```python
from build123d import *

# Parameters (mm, degrees)
F1_DEPTH = 15
F2_R     = 37.5
F3_DEPTH = 50
F4_R     = 7.5
F5_DEPTH = 40
F7_DEPTH = 50


with BuildPart() as f1:
    # F0 (on Front) → F1 (new body, symmetric)
    with BuildSketch(Plane.XZ):
        Polygon((-25, 200), (-75, 200), (-17.5, -30), (15, -30), (187.5, 200), (112.5, 200), (9.375, 62.5), align=None)
    extrude(amount=F1_DEPTH, both=True)

    # F2 (on Front) → F3 (join, symmetric)
    with BuildSketch(Plane.XZ):
        Circle(F2_R)
    extrude(amount=F3_DEPTH, both=True)

    # F4 (on face) → F5 (join)
    with BuildSketch(Plane.XZ.offset(50)):
        Circle(F4_R)
    extrude(amount=F5_DEPTH)

    # F6 (on Top) → F7 (cut, symmetric)
    with BuildSketch(Plane.XY):
        Polygon((-20, -79.282032), (-20, -90), (20, -90), align=None)
    extrude(amount=F7_DEPTH, both=True, mode=Mode.SUBTRACT)


solid = f1.part
```
Build history of the part. All positions in model axes, mm. A direction names the side the tool comes from. Coordinates: 2 decimals unless noted, no trailing zeros. Order: outer loops, then holes, each group sorted by start corner. A loop starts at its lowest first (then second) coordinate and runs counter-clockwise, first axis right, second up.
Item 1: Mould opens along X. For faces 1 (the flat face through (111.45, -0.21, 98.6)), 2 (the flat face through (54, -15, 101)), 3 (the flat face through (-7.572, -0.21, 130.288)) say: released by +X, released by -X, zero draft, split by the parting line, or undercut.
Filled in:
face 1: released by +X
face 2: zero draft
face 3: undercut
Item 2: Tool access for faces 4 (the flat face through (-1, 50, 1)), 5 (the flat face through (61.66, -0.21, 132.21)), 6 (the cylindrical face through (7.154, -68.069, 2.253)), 7 (the cylindrical face through (-8.13, -0.7, -36.61)): list every direction of +Z, -Z, +X, -X, +Y, -Y with a clear straight run to the whole face (end or side of a thin tool).
Filled in:
face 4: +Z, -Z, +X, -X, +Y
face 5: +Z, +Y, -Y
face 6: -Y
face 7: none
Item 3: Saw through at B-B on x = 29. List the corners of the cut face in (y, z), then the cut area to 3 significant figures.
Filled in:
outline: (-50, -23.77) - (50, -23.77) - (50, 23.77) - (15, 23.77) - (15, 88.67) - (-15, 88.67) - (-15, 23.77) - (-50, 23.77) - close
area: 6,700 mm2
Item 4: Drill centre lines: L1, parallel to Y at x = 99, z = 96; L2, parallel to X at y = -1, z = -25.5; L3, parallel to Z at x = -3, y = 21. Where is each one in solid material? Low to high.
Filled in:
L1: y = -15 to 15
L2: x = -27.5 to 27.5
L3: z = -37.38 to 37.38
Item 5: Drop flat-ended pins along their axis: pin 1 Ø5 at (x, y) = (31, -50) entering from +Z; pin 2 Ø6 at (y, z) = (7, 33) entering from -X; pin 3 Ø8 at (y, z) = (-21.5, 92.5) entering from -X; pin 4 Ø3 at (x, y) = (155.5, 15) entering from -Z. Give the stop position or say it passes through.
Filled in:
pin 1: stops at z = 24.37
pin 2: stops at x = -34
pin 3: passes through
pin 4: stops at z = 155.33
Item 6: Saw through at D-D on y = 29.5. List the corners of the cut face in (x, z).
Filled in:
outline: circle Ø75 at (0, 0)
Item 7: Saw through at A-A on z = 90.5. List the corners of the cut face in (x, y) (3 decimals), then the cut area to 3 significant figures.
Filled in:
outline: (-47.625, -15) - (2.375, -15) - (2.375, 15) - (-47.625, 15) - close; (30.375, -15) - (105.375, -15) - (105.375, 15) - (30.375, 15) - close
area: 3,750 mm2
Item 8: Saw through at C-C on z = 31.5. List the corners of the cut face in (x, y) (3 decimals).
Filled in:
outline: (-32.875, -15) - (-20.347, -15) - (-20.347, -50) - (20.347, -50) - (20.347, -15) - (61.125, -15) - (61.125, 15) - (20.347, 15) - (20.347, 50) - (-20.347, 50) - (-20.347, 15) - (-32.875, 15) - close
